```python
from build123d import *

# Parameters (mm, degrees)
SKETCH_1_W      = 7.1
SKETCH_1_H      = 6.6
EXTRUDE_1_DEPTH = 3
FILLET_1_R      = 0.5
SKETCH_2_W      = 0.5
SKETCH_2_H      = 3
EXTRUDE_2_DEPTH = 2


with BuildPart() as part:
    # 草图1 → 凸台-拉伸1 (new body)
    with BuildSketch(Plane(origin=(0, 0, 0), x_dir=(1, 0, 0), z_dir=(0, 1, 0))):
        Rectangle(SKETCH_1_W, SKETCH_1_H)
    extrude(amount=EXTRUDE_1_DEPTH)

    # 圆角1
    fillet_1_edges = [part.edges().sort_by_distance(p)[0] for p in [
        (3.55, 1.5, 3.3),
        (-3.55, 1.5, 3.3),
        (-3.55, 1.5, -3.3),
        (3.55, 1.5, -3.3),
    ]]
    fillet(fillet_1_edges, radius=FILLET_1_R)

    # 草图2 → 凸台-拉伸2 (add)
    with BuildSketch(Plane.XZ):
        with Locations((-3.55, 0)):
            Rectangle(SKETCH_2_W, SKETCH_2_H)
        with Locations((3.55, 0)):
            Rectangle(SKETCH_2_W, SKETCH_2_H)
    extrude(amount=-EXTRUDE_2_DEPTH)


solid = part.part
```
Design review of the part built by this model. Coordinates are the model's own, in mm. Round coordinates to 2 decimals unless told otherwise and drop trailing zeros. Write each loop counter-clockwise with the first axis right and the second up, starting at its lowest first coordinate (ties: lowest second). Pieces come first, ordered by that corner, then holes. Notation, with made-up numbers: (-9, -36) -> (-2, -36) arc R6 cw to (-2, -32) -> close; hole circle Ø11 at (19.25, 78). An arc over 180 degrees is marked (long way). Write item = value, one per line. Start each with the question number.
1) Take a section at A-A, the plane y = 2.45. State the section outline as (x, z) points, plus the area to 3 significant figures.
2) Take a section at C-C, the plane y = 1.15. State the section outline as (x, z) points.
3) Take a section at D-D, the plane z = 1.75. State the section outline as (x, y) points.
4) Take a section at B-B, the plane z = 1. State the section outline as (x, y) points.
5) Wall thickness on probe 1 along X at (y, z) = (2.4, -2.5); probe 2 along X at (y, z) = (0.5, 3): over which ranges is each line inside the solid? List them lowest first. Write a range as from..to.
Results list:
q1.outline = (-3.55, -2.8) arc R0.5 ccw to (-3.05, -3.3) -> (3.05, -3.3) arc R0.5 ccw to (3.55, -2.8) -> (3.55, 2.8) arc R0.5 ccw to (3.05, 3.3) -> (-3.05, 3.3) arc R0.5 ccw to (-3.55, 2.8) -> close
q1.area = 46.6 mm²
q2.outline = (-3.8, -1.5) -> (-3.55, -1.5) -> (-3.55, -2.8) arc R0.5 ccw to (-3.05, -3.3) -> (3.05, -3.3) arc R0.5 ccw to (3.55, -2.8) -> (3.55, -1.5) -> (3.8, -1.5) -> (3.8, 1.5) -> (3.55, 1.5) -> (3.55, 2.8) arc R0.5 ccw to (3.05, 3.3) -> (-3.05, 3.3) arc R0.5 ccw to (-3.55, 2.8) -> (-3.55, 1.5) -> (-3.8, 1.5) -> close
q3.outline = (-3.55, 0) -> (3.55, 0) -> (3.55, 3) -> (-3.55, 3) -> close
q4.outline = (-3.8, 0) -> (3.8, 0) -> (3.8, 2) -> (3.55, 2) -> (3.55, 3) -> (-3.55, 3) -> (-3.55, 2) -> (-3.8, 2) -> close
q5.probe_1 = -3.55..3.55
q5.probe_2 = -3.51..3.51
